Design review of the part built by this model. Coordinates are the model's own, in mm. Give positions to 0.01 mm unless a question says otherwise; leave off trailing zeros. Use a Markdown table: item, result. Add a question column.
(1) Add section A-A, the plane z = -158.5. State how many separate pieces and enclosed holes the cut face has, then the cut area to 3 significant figures.
(2) Insertion check: pin 1 Ø8 at (x, z) = (11, -181.5) entering from +Y; pin 2 Ø2.5 at (y, z) = (14, -220) entering from +X; pin 3 Ø0.7 at (x, z) = (7, -159.5) entering from +Y. Each pin has a flat end and moves straight along its axis. Give the tip position at first contact, or say it passes through.
(3) For probe 1 along Y at (x, z) = (-9.5, -61.5); probe 2 along X at (y, z) = (13.5, -68.5); probe 3 along Y at (x, z) = (-9, -217.5), list the stretches that pass through material, from the lowest coordinate up.
```python
from build123d import *

# Parameters (mm, degrees)
SKETCH1_R      = 3.4
EXTRUDE1_DEPTH = 300


with BuildPart() as part:
    # Sketch1 → Extrude1 (new body)
    with BuildSketch(Plane.XY):
        with BuildLine():
            Line((-13.552721419, -20), (-17.142397126, -20))
            ThreePointArc((-17.142397126, -20), (-18.235954402, -19.782477933), (-19.163027496, -19.163027496))
            ThreePointArc((-19.163027496, -19.163027496), (-19.782477933, -18.235954402), (-20, -17.142397126))
            Line((-20, -17.142397126), (-20, -13.552721419))
            Line((-20, -13.552721419), (-20, -5.540330257))
            ThreePointArc((-20, -5.540330257), (-19.566421306, -4.493578694), (-18.519669743, -4.06))
            Line((-18.519669743, -4.06), (-17.804849126, -4.06))
            ThreePointArc((-17.804849126, -4.06), (-16.486201663, -4.606201663), (-15.94, -5.924849126))
            Line((-15.94, -5.924849126), (-15.94, -7.280726922))
            Line((-15.94, -7.280726922), (-16.7, -7.280726922))
            Line((-16.7, -7.280726922), (-16.7, -9.015))
            ThreePointArc((-16.7, -9.015), (-16.328025612, -9.913025612), (-15.43, -10.285))
            Line((-15.43, -10.285), (-13.053775012, -10.285))
            ThreePointArc((-13.053775012, -10.285), (-12.65158934, -10.205000296), (-12.310632791, -9.977180413))
            Line((-12.310632791, -9.977180413), (-9.431242789, -7.097790411))
            ThreePointArc((-9.431242789, -7.097790411), (-8.401572221, -5.556779505), (-8.04, -3.739033201))
            Line((-8.04, -3.739033201), (-8.04, 3.739033201))
            ThreePointArc((-8.04, 3.739033201), (-8.401572221, 5.556779505), (-9.431242789, 7.097790411))
            Line((-9.431242789, 7.097790411), (-12.357777413, 10.024325035))
            ThreePointArc((-12.357777413, 10.024325035), (-12.646514194, 10.217252784), (-12.987102448, 10.285))
            Line((-12.987102448, 10.285), (-15.363327437, 10.285))
            ThreePointArc((-15.363327437, 10.285), (-16.30849767, 9.89349767), (-16.7, 8.948327437))
            Line((-16.7, 8.948327437), (-16.7, 7.280726922))
            Line((-16.7, 7.280726922), (-15.94, 7.280726922))
            Line((-15.94, 7.280726922), (-15.94, 5.924849126))
            ThreePointArc((-15.94, 5.924849126), (-16.486201663, 4.606201663), (-17.804849126, 4.06))
            Line((-17.804849126, 4.06), (-18.519669743, 4.06))
            ThreePointArc((-18.519669743, 4.06), (-19.566421306, 4.493578694), (-20, 5.540330257))
            Line((-20, 5.540330257), (-20, 12.563650804))
            Line((-20, 12.563650804), (-20, 16.832984559))
            ThreePointArc((-20, 16.832984559), (-19.072402654, 19.072402654), (-16.832984559, 20))
            Line((-16.832984559, 20), (-10, 20))
            ThreePointArc((-10, 20), (11.213203436, 11.213203436), (20, -10))
            Line((20, -10), (20, -16.832984559))
            ThreePointArc((20, -16.832984559), (19.072402654, -19.072402654), (16.832984559, -20))
            Line((16.832984559, -20), (12.563650804, -20))
            Line((12.563650804, -20), (5.540330257, -20))
            ThreePointArc((5.540330257, -20), (4.493578694, -19.566421306), (4.06, -18.519669743))
            Line((4.06, -18.519669743), (4.06, -17.804849126))
            ThreePointArc((4.06, -17.804849126), (4.606201663, -16.486201663), (5.924849126, -15.94))
            Line((5.924849126, -15.94), (7.280726922, -15.94))
            Line((7.280726922, -15.94), (7.280726922, -16.7))
            Line((7.280726922, -16.7), (8.948327437, -16.7))
            ThreePointArc((8.948327437, -16.7), (9.89349767, -16.30849767), (10.285, -15.363327437))
            Line((10.285, -15.363327437), (10.285, -12.987102448))
            ThreePointArc((10.285, -12.987102448), (10.217252784, -12.646514194), (10.024325035, -12.357777413))
            Line((10.024325035, -12.357777413), (7.097790411, -9.431242789))
            ThreePointArc((7.097790411, -9.431242789), (5.556779505, -8.401572221), (3.739033201, -8.04))
            Line((3.739033201, -8.04), (-3.739033201, -8.04))
            ThreePointArc((-3.739033201, -8.04), (-5.556779505, -8.401572221), (-7.097790411, -9.431242789))
            Line((-7.097790411, -9.431242789), (-9.977180413, -12.310632791))
            ThreePointArc((-9.977180413, -12.310632791), (-10.205000296, -12.65158934), (-10.285, -13.053775012))
            Line((-10.285, -13.053775012), (-10.285, -15.43))
            ThreePointArc((-10.285, -15.43), (-9.913025612, -16.328025612), (-9.015, -16.7))
            Line((-9.015, -16.7), (-7.280726922, -16.7))
            Line((-7.280726922, -16.7), (-7.280726922, -15.94))
            Line((-7.280726922, -15.94), (-5.924849126, -15.94))
            ThreePointArc((-5.924849126, -15.94), (-4.606201663, -16.486201663), (-4.06, -17.804849126))
            Line((-4.06, -17.804849126), (-4.06, -18.519669743))
            ThreePointArc((-4.06, -18.519669743), (-4.493578694, -19.566421306), (-5.540330257, -20))
            Line((-5.540330257, -20), (-13.552721419, -20))
        make_face()
        Circle(SKETCH1_R, mode=Mode.SUBTRACT)
        with BuildLine():
            Line((-11.925, -17.705), (-11.925, -13.195))
            ThreePointArc((-11.925, -13.195), (-12.296974388, -12.296974388), (-13.195, -11.925))
            Line((-13.195, -11.925), (-17.705, -11.925))
            ThreePointArc((-17.705, -11.925), (-18.150477272, -12.109522728), (-18.335, -12.555))
            Line((-18.335, -12.555), (-18.335, -15.535))
            ThreePointArc((-18.335, -15.535), (-17.514898987, -17.514898987), (-15.535, -18.335))
            Line((-15.535, -18.335), (-12.555, -18.335))
            ThreePointArc((-12.555, -18.335), (-12.109522728, -18.150477272), (-11.925, -17.705))
        make_face(mode=Mode.SUBTRACT)
        with BuildLine():
            Line((7.679270597, 0), (7.679270597, -3.378303798))
            ThreePointArc((7.679270597, -3.378303798), (8.040842817, -5.196050101), (9.070513386, -6.737061008))
            Line((9.070513386, -6.737061008), (12.400776329, -10.067323951))
            ThreePointArc((12.400776329, -10.067323951), (12.647338074, -10.232071242), (12.938177482, -10.289922797))
            Line((12.938177482, -10.289922797), (17.586072346, -10.289922797))
            ThreePointArc((17.586072346, -10.289922797), (18.12803226, -10.062726187), (18.345962028, -9.516973987))
            ThreePointArc((18.345962028, -9.516973987), (16.406061612, 0.317305248), (11.165061741, 8.861787798))
            ThreePointArc((11.165061741, 8.861787798), (10.619514718, 9.11583304), (10.060274233, 8.893548045))
            Line((10.060274233, 8.893548045), (6.444636983, 5.277910795))
            ThreePointArc((6.444636983, 5.277910795), (6.225426758, 4.812198006), (6.353269463, 4.313602211))
            ThreePointArc((6.353269463, 4.313602211), (7.34028856, 2.256404387), (7.679270597, 0))
        make_face(mode=Mode.SUBTRACT)
        with BuildLine():
            Line((17.720077203, -11.939922797), (13.210077203, -11.939922797))
            ThreePointArc((13.210077203, -11.939922797), (12.312051591, -12.311897185), (11.940077203, -13.209922797))
            Line((11.940077203, -13.209922797), (11.940077203, -17.719922797))
            ThreePointArc((11.940077203, -17.719922797), (12.124599931, -18.165400069), (12.570077203, -18.349922797))
            Line((12.570077203, -18.349922797), (15.550077203, -18.349922797))
            ThreePointArc((15.550077203, -18.349922797), (17.52997619, -17.529821784), (18.350077203, -15.549922797))
            Line((18.350077203, -15.549922797), (18.350077203, -12.569922797))
            ThreePointArc((18.350077203, -12.569922797), (18.165554475, -12.124445525), (17.720077203, -11.939922797))
        make_face(mode=Mode.SUBTRACT)
        with BuildLine():
            Line((-13.209922797, 11.940077203), (-17.719922797, 11.940077203))
            ThreePointArc((-17.719922797, 11.940077203), (-18.165400069, 12.124599931), (-18.349922797, 12.570077203))
            Line((-18.349922797, 12.570077203), (-18.349922797, 15.550077203))
            ThreePointArc((-18.349922797, 15.550077203), (-17.529821784, 17.52997619), (-15.549922797, 18.350077203))
            Line((-15.549922797, 18.350077203), (-12.569922797, 18.350077203))
            ThreePointArc((-12.569922797, 18.350077203), (-12.124445525, 18.165554475), (-11.939922797, 17.720077203))
            Line((-11.939922797, 17.720077203), (-11.939922797, 13.210077203))
            ThreePointArc((-11.939922797, 13.210077203), (-12.311897185, 12.312051591), (-13.209922797, 11.940077203))
        make_face(mode=Mode.SUBTRACT)
        with BuildLine():
            Line((8.893548045, 10.060274233), (5.277910795, 6.444636983))
            ThreePointArc((5.277910795, 6.444636983), (4.812198006, 6.225426758), (4.313602211, 6.353269463))
            ThreePointArc((4.313602211, 6.353269463), (2.256404387, 7.34028856), (0, 7.679270597))
            Line((0, 7.679270597), (-3.378303798, 7.679270597))
            ThreePointArc((-3.378303798, 7.679270597), (-5.196050101, 8.040842817), (-6.737061008, 9.070513386))
            Line((-6.737061008, 9.070513386), (-10.067323951, 12.400776329))
            ThreePointArc((-10.067323951, 12.400776329), (-10.232071242, 12.647338074), (-10.289922797, 12.938177482))
            Line((-10.289922797, 12.938177482), (-10.289922797, 17.586072346))
            ThreePointArc((-10.289922797, 17.586072346), (-10.062726187, 18.12803226), (-9.516973987, 18.345962028))
            ThreePointArc((-9.516973987, 18.345962028), (0.317305248, 16.406061612), (8.861787798, 11.165061741))
            ThreePointArc((8.861787798, 11.165061741), (9.11583304, 10.619514718), (8.893548045, 10.060274233))
        make_face(mode=Mode.SUBTRACT)
    extrude(amount=-EXTRUDE1_DEPTH)


solid = part.part
```
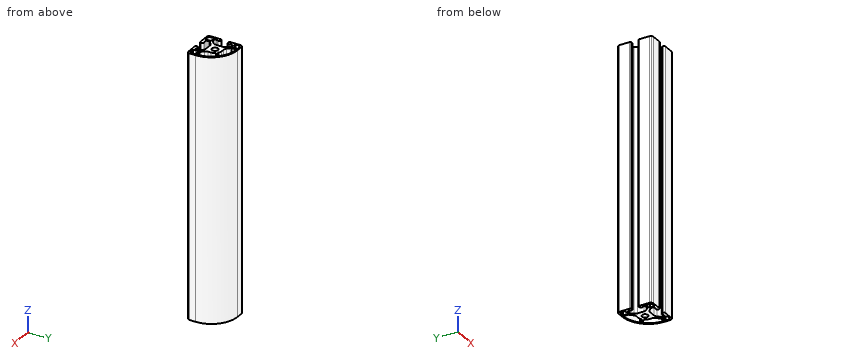
Established:
| question | item | result |
|---|---|---|
| 1 | separate pieces | 1 |
| 1 | enclosed holes | 6 |
| 1 | area | 588 mm^2 |
| 2 | pin 1 | y = 14.72 |
| 2 | pin 2 | x = 9.56 |
| 2 | pin 3 | y = 14.96 |
| 3 | probe 1 | -20 to -16.6, -11.83 to -7.17, 7.17 to 11.83, 18.35 to 20 |
| 3 | probe 2 | -20 to -18.35, -11.94 to -10.29, 5.86 to 8.65 |
| 3 | probe 3 | -20 to -16.7, -11.33 to -6.6, 6.6 to 11.33, 18.33 to 19.98 |
